The listing builds one solid part. Answer for the finished solid, in the listing's coordinates (mm). Face numbers are marked on the shaded views. Give positions to 0.01 mm unless a question says otherwise; leave off trailing zeros. Write each loop counter-clockwise with the first axis right and the second up, starting at its lowest first coordinate (ties: lowest second). Pieces come first, ordered by that corner, then holes. Notation, with made-up numbers: (41, 30.5) - (92, 30.5) arc R18 cw to (92, 37.5) - close; hole circle Ø9 at (-37.75, -10). An arc over 180 degrees is marked (long way). Return JSON: item names as keys, results as strings.
from build123d import *

# Parameters (mm, degrees)
SKETCH1_R                       = 60.96
BILLET_DEPTH                    = 12.7
SKETCH4_R                       = 0.7493
FIRST_KEROSENE_OUTLET_DEPTH     = 88.140881336
PRIMARY_HOLES_COUNT             = 6
SECOND_START                    = -12.7
SECOND_RING_OUTLINE_R           = 0.7493
SECOND_RING_DEPTH               = 12.7
THIRD_START                     = -12.7
THIRD_RING_OUTLINE_R            = 0.7493
THIRD_RING_DEPTH                = 12.7
SKETCH18_RX                     = 46.67504
SKETCH18_RY                     = 22.225
KEROSENE_WELL_DEPTH             = 9.3218
SKETCH17_R                      = 6.35
BOSS_EXTRUDE1_DEPTH             = 2.54
BOSS_EXTRUDE1_DIRECTION_2_REACH = 89.141
SKETCH21_R                      = 6.35
CUT_EXTRUDE1_DEPTH              = 2.54
CUT_EXTRUDE2_DEPTH              = 2.54
SKETCH15_R                      = 59.69
SKETCH15_R_2                    = 57.15
CUT_EXTRUDE3_DEPTH              = 1.778
F_1_8_0_125_DIAMETER_HOLE2_D    = 3.175
SKETCH31_R                      = 7.24947448
SKETCH31_R_2                    = 6.200396603
CUT_EXTRUDE4_DEPTH              = 1.778


# Read off the part's stored shape, not the designer's step: Second ring, Third Ring
with BuildPart() as part:
    # Sketch1 → Billet (new body)
    with BuildSketch(Plane(origin=(0, 0, 0), x_dir=(1, 0, 0), z_dir=(0, 1, 0))):
        with Locations(Location((0, 0, 0), (0, 0, 270))):
            Circle(SKETCH1_R)
    extrude(amount=-BILLET_DEPTH)

    # Sketch4 → First Kerosene Outlet (cut, symmetric)
    with BuildSketch(Plane(origin=(0, -12.7, 0), x_dir=(1, 0, 0), z_dir=(0, 1, 0))):
        with Locations(Location((8.9916, 0, 0), (0, 0, 270))):
            Circle(SKETCH4_R)
        with Locations(Location((13.4874, 0, 0), (0, 0, 270))):
            Circle(SKETCH4_R)
        with Locations(Location((17.9832, 0, 0), (0, 0, 270))):
            Circle(SKETCH4_R)
    first_kerosene_outlet = extrude(amount=FIRST_KEROSENE_OUTLET_DEPTH, both=True, mode=Mode.SUBTRACT)

    # Primary Holes: First Kerosene Outlet ×6 about axis
    primary_holes_axis = Axis((0, 0, 0), (0, 1, 0))
    for i in range(1, PRIMARY_HOLES_COUNT):
        add(first_kerosene_outlet.rotate(primary_holes_axis, i * 360 / PRIMARY_HOLES_COUNT), mode=Mode.SUBTRACT)

    # Second ring outline → Second ring (cut)
    with BuildSketch(Plane(origin=(0, 0, 0), x_dir=(1, 0, 0), z_dir=(0, 1, 0)).offset(SECOND_START)):
        with Locations((11.680431031, 6.7437)):
            Circle(SECOND_RING_OUTLINE_R)
        with Locations((0, 13.4874)):
            Circle(SECOND_RING_OUTLINE_R)
        with Locations((-11.680431031, 6.7437)):
            Circle(SECOND_RING_OUTLINE_R)
        with Locations((-11.680431031, -6.7437)):
            Circle(SECOND_RING_OUTLINE_R)
        with Locations((0, -13.4874)):
            Circle(SECOND_RING_OUTLINE_R)
        with Locations((11.680431031, -6.7437)):
            Circle(SECOND_RING_OUTLINE_R)
    extrude(amount=SECOND_RING_DEPTH, mode=Mode.SUBTRACT)

    # Third Ring outline → Third Ring (cut)
    with BuildSketch(Plane(origin=(0, 0, 0), x_dir=(1, 0, 0), z_dir=(0, 1, 0)).offset(THIRD_START)):
        with Locations((17.370437319, 4.654394652)):
            Circle(THIRD_RING_OUTLINE_R)
        with Locations((15.573908041, 8.9916)):
            Circle(THIRD_RING_OUTLINE_R)
        with Locations((12.716042667, 12.716042667)):
            Circle(THIRD_RING_OUTLINE_R)
        with Locations((4.654394652, 17.370437319)):
            Circle(THIRD_RING_OUTLINE_R)
        with Locations((0, 17.9832)):
            Circle(THIRD_RING_OUTLINE_R)
        with Locations((-4.654394652, 17.370437319)):
            Circle(THIRD_RING_OUTLINE_R)
        with Locations((-12.716042667, 12.716042667)):
            Circle(THIRD_RING_OUTLINE_R)
        with Locations((-15.573908041, 8.9916)):
            Circle(THIRD_RING_OUTLINE_R)
        with Locations((-17.370437319, 4.654394652)):
            Circle(THIRD_RING_OUTLINE_R)
        with Locations((-17.370437319, -4.654394652)):
            Circle(THIRD_RING_OUTLINE_R)
        with Locations((-15.573908041, -8.9916)):
            Circle(THIRD_RING_OUTLINE_R)
        with Locations((-12.716042667, -12.716042667)):
            Circle(THIRD_RING_OUTLINE_R)
        with Locations((-4.654394652, -17.370437319)):
            Circle(THIRD_RING_OUTLINE_R)
        with Locations((0, -17.9832)):
            Circle(THIRD_RING_OUTLINE_R)
        with Locations((4.654394652, -17.370437319)):
            Circle(THIRD_RING_OUTLINE_R)
        with Locations((12.716042667, -12.716042667)):
            Circle(THIRD_RING_OUTLINE_R)
        with Locations((15.573908041, -8.9916)):
            Circle(THIRD_RING_OUTLINE_R)
        with Locations((17.370437319, -4.654394652)):
            Circle(THIRD_RING_OUTLINE_R)
    extrude(amount=THIRD_RING_DEPTH, mode=Mode.SUBTRACT)

    # Sketch18 → Kerosene Well (cut)
    with BuildSketch(Plane(origin=(0, 0, 0), x_dir=(1, 0, 0), z_dir=(0, 1, 0))):
        with Locations(Location((0, 0), (0, 0, -180))):
            Ellipse(SKETCH18_RX, SKETCH18_RY)
    extrude(amount=-KEROSENE_WELL_DEPTH, mode=Mode.SUBTRACT)

    # Sketch17 → Boss-Extrude1 (add)
    with BuildSketch(Plane(origin=(0, 0, 0), x_dir=(1, 0, 0), z_dir=(0, 1, 0))):
        with Locations(Location((0, 0, 0), (0, 0, 270))):
            Circle(SKETCH17_R)
    extrude(amount=BOSS_EXTRUDE1_DEPTH)

    # Sketch17 → Boss-Extrude1 direction 2 (add, up to next)
    with BuildSketch(Plane(origin=(0, 0, 0), x_dir=(1, 0, 0), z_dir=(0, 1, 0)), mode=Mode.PRIVATE) as boss_extrude1_direction_2_sk1:
        with Locations(Location((0, 0, 0), (0, 0, 270))):
            Circle(SKETCH17_R)
    boss_extrude1_direction_2_tool1 = extrude(boss_extrude1_direction_2_sk1.sketch, amount=-BOSS_EXTRUDE1_DIRECTION_2_REACH, mode=Mode.PRIVATE) - part.part
    add(boss_extrude1_direction_2_tool1.solids().sort_by_distance((0, 0, 0))[0])

    # Sketch21 → Cut-Extrude1 (cut)
    with BuildSketch(Plane(origin=(0, 2.54, 0), x_dir=(1, 0, 0), z_dir=(0, 1, 0))):
        with Locations(Location((0, 0, 0), (0, 0, 270))):
            Circle(SKETCH21_R)
    extrude(amount=-CUT_EXTRUDE1_DEPTH, mode=Mode.SUBTRACT)

    # Sketch24 → Cut-Extrude2 (cut)
    with BuildSketch(Plane(origin=(0, 0, 0), x_dir=(1, 0, 0), z_dir=(0, 1, 0))):
        with BuildLine():
            Line((-15.732765962, 20.924382105), (-21.799630657, 31.4325))
            ThreePointArc((-21.799630657, 31.4325), (-20.6375, 35.769630657), (-16.300369343, 34.6075))
            Line((-16.300369343, 34.6075), (-8.915091663, 21.81582383))
            add(Edge.make_bspline(
                [(-8.915091663, 21.81582383), (-12.395027666, 21.493390748), (-15.732765962, 20.924382105)],
                knots=[4.904573252, 4.904573252, 4.904573252, 5.056192247, 5.056192247, 5.056192247], degree=2, weights=[1, 0.997127836, 1]))
        make_face()
    extrude(amount=-CUT_EXTRUDE2_DEPTH, mode=Mode.SUBTRACT)

    # Sketch15 → Cut-Extrude3 (cut)
    with BuildSketch(Plane(origin=(0, -12.7, 0), x_dir=(1, 0, 0), z_dir=(0, 1, 0))):
        with Locations(Location((0, 0, 0), (0, 0, 270))):
            Circle(SKETCH15_R)
        with Locations(Location((0, 0, 0), (0, 0, 270))):
            Circle(SKETCH15_R_2, mode=Mode.SUBTRACT)
    extrude(amount=CUT_EXTRUDE3_DEPTH, mode=Mode.SUBTRACT)

    # 1/8 (0.125) Diameter Hole2 (through all)
    with Locations(Plane(origin=(19.05, 0, -33.02), x_dir=(0, 0, 1), z_dir=(0, 1, 0))):
        with Locations((0, 0)):
            Hole(F_1_8_0_125_DIAMETER_HOLE2_D / 2)

    # Sketch31 → Cut-Extrude4 (cut)
    with BuildSketch(Plane(origin=(0, 0, 0), x_dir=(1, 0, 0), z_dir=(0, 1, 0))):
        with Locations(Location((19.05, 33.02, 0), (0, 0, 270))):
            Circle(SKETCH31_R)
        with Locations(Location((19.05, 33.02, 0), (0, 0, 270))):
            Circle(SKETCH31_R_2, mode=Mode.SUBTRACT)
    extrude(amount=-CUT_EXTRUDE4_DEPTH, mode=Mode.SUBTRACT)


solid = part.part
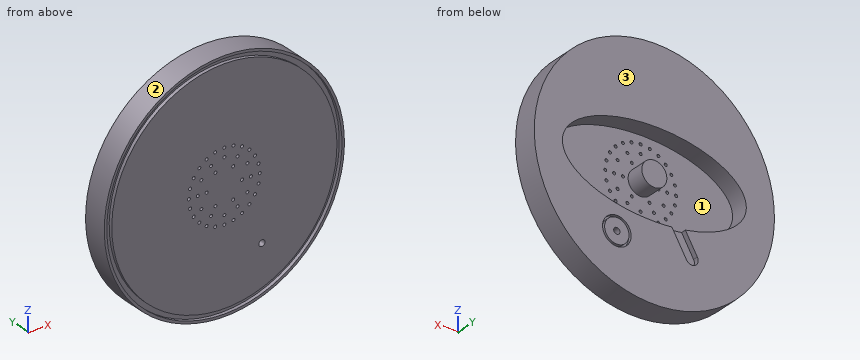
Item 1: A cutting plane is placed at A-A on z = -33.02. Determine the outline of the cut face in (x, y) (1 decimal).
Answer below:
{"outline": "(-51.2, -12.7) - (-49.7, -12.7) - (-49.7, -10.9) - (-46.6, -10.9) - (-46.6, -12.7) - (17.5, -12.7) - (17.5, 0) - (12.8, 0) - (12.8, -1.8) - (11.8, -1.8) - (11.8, 0) - (-15.4, 0) - (-15.4, -2.5) - (-22.2, -2.5) - (-22.2, 0) - (-51.2, 0) - close; (20.6, -12.7) - (46.6, -12.7) - (46.6, -10.9) - (49.7, -10.9) - (49.7, -12.7) - (51.2, -12.7) - (51.2, 0) - (26.3, 0) - (26.3, -1.8) - (25.3, -1.8) - (25.3, 0) - (20.6, 0) - close"}
Item 2: Consider L1, parallel to Z at x = 2, y = -6.5; L2, parallel to X at y = -11.75, z = -20.5; L3, parallel to Y at x = 29, z = 1. Determine where each line is inside the solid, lowest interval first.
Answer below:
{"L1": "z = -60.93 to -22.2, -6.03 to 6.03, 22.2 to 60.93", "L2": "x = -57.41 to -56.06, -53.35 to 53.35, 56.06 to 57.41", "L3": "y = -12.7 to -9.32"}
Item 3: Flat-ended cylindrical pins translate along their axes: P1, Ø4, axis at x = 46, y = -3, coming from the -Z side; P2, Ø1.3, axis at x = 4.65, z = -17.37, coming from the +Y side; P3, Ø1.5, axis at x = 40.5, y = -6, coming from the -Z side; P4, Ø4, axis at y = -8.5, z = 2, coming from the +X side. Find the tip coordinate at first contact, or state that the pin passes through.
Answer below:
{"P1": "stops at z = -42.19", "P2": "passes through", "P3": "stops at z = -46.22", "P4": "stops at x = 60.96"}
Item 4: A cutting plane is placed at C-C on z = 30. Determine the outline of the cut face in (x, y).
Answer below:
{"outline": "(-53.07, -12.7) - (-51.6, -12.7) - (-51.6, -10.92) - (-48.64, -10.92) - (-48.64, -12.7) - (48.64, -12.7) - (48.64, -10.92) - (51.6, -10.92) - (51.6, -12.7) - (53.07, -12.7) - (53.07, 0) - (-53.07, 0) - close"}
Item 5: A cutting plane is placed at B-B on y = -6.25. Give the number of separate pieces and of enclosed holes in the cut face, then the cut area to 3 significant figures.
Answer below:
{"separate pieces": "2", "enclosed holes": "2", "area": "8,530 mm²"}
Item 6: The mould has two halves that part along X. Classify the marked faces 1, 2 and 3: +X half, -X half, draft (parallel to the pull), parting line (faces both ways), or undercut.
Answer below:
{"face 1": "undercut", "face 2": "parting line", "face 3": "draft"}
